from build123d import *

# Parameters (mm, degrees)
SKETCH1_R           = 3
BOSS_EXTRUDE1_DEPTH = 120
FILLET1_R           = 1


with BuildPart() as part:
    # Sketch1 → Boss-Extrude1 (new body)
    with BuildSketch(Plane.XY):
        Circle(SKETCH1_R)
    extrude(amount=BOSS_EXTRUDE1_DEPTH)

    # Sketch4 → Revolve2 (revolve)
    with BuildSketch(Plane(origin=(0, 0, 0), x_dir=(1, 0, 0), z_dir=(0, 1, 0)), mode=Mode.PRIVATE) as revolve2_sk:
        Polygon((3, -120), (0, -125.982943807), (0, -120), align=None)
    revolve(revolve2_sk.sketch.rotate(Axis((0, 0, 147.90647938), (0, 0, -1)), 180), axis=Axis((0, 0, 147.90647938), (0, 0, -1)))

    # Fillet1
    fillet1_edges = [part.edges().sort_by_distance(p)[0] for p in [
        (-3, 0, 0),
    ]]
    fillet(fillet1_edges, radius=FILLET1_R)


solid = part.part
The listing builds one solid part. Answer for the finished solid, in the listing's coordinates (mm). Round coordinates to 2 decimals unless told otherwise and drop trailing zeros. Order: outer loops, then holes, each group sorted by start corner. A loop starts at its lowest first (then second) coordinate and runs counter-clockwise, first axis right, second up. Notation, with made-up numbers: (65, 47.25) -> (79, 47.25) arc R18 cw to (79, 72.25) -> close; hole circle Ø8 at (23.25, 68). An arc over 180 degrees is marked (long way). Put each result on its own line as item: value.
Q1. Each of these flat-tipped pins is pushed along its axis until it touches: P1, Ø2, axis at x = -0.5, y = 1.5, coming from the +Z side; P2, Ø3, axis at x = 1.5, z = 76.5, coming from the -Y side; P3, Ø3, axis at x = 1.5, y = -0.5, coming from the +Z side. Where does it stop, or does it pass through?
Results list:
P1: z = 124.82
P2: y = -3
P3: z = 125.82
Q2. Section A-A, the plane z = 113 is taken. Write down the section's boundary in (x, y), and give its area (3 significant figures).
Results list:
outline: circle Ø6 at (0, 0)
area: 28.3 mm^2
Q3. Consider line 1 along Y through (x, z) = (0.35, 44); line 2 along X through (y, z) = (-0.1, 77.5); line 3 along Z through (x, y) = (2.4, 1.1). Determine where each line is inside the solid, lowest interval first.
Results list:
line 1: -2.98 to 2.98
line 2: -3 to 3
line 3: 0.23 to 120.72
